Geometry: final body of the model. Coordinates: model frame, mm. Face numbers are marked on the shaded views. A direction names the side the tool comes from. Give positions to 0.01 mm unless a question says otherwise; leave off trailing zeros. Loops run counter-clockwise (first coordinate to the right, second up) from the corner with the lowest first, then second, coordinate; pieces in that order, holes last. Notation, with made-up numbers: (11.5, -32.5) -> (40.5, -32.5) arc R25 cw to (40.5, -0.5) -> close; hole circle Ø1 at (71.5, 68.25). An arc over 180 degrees is marked (long way). Answer in a Markdown table with one row per item. Add a question column.
1) Line query: line 1 (Y direction, x = -0.5, z = -9); line 2 (Z direction, x = 24, y = 9); line 3 (Z direction, x = 7, y = -8). Output: solid intervals per line, ascending. Write a range as from..to.
2) First-contact query: P1, Ø1, axis at x = -3.5, z = -2, coming from the -Y side; P2, Ø12, axis at y = 3.5, z = -1, coming from the +X side; P3, Ø6.5, axis at x = 25, z = 0, coming from the -Y side. Flat tips, straight axial feed; report the tip coordinate or a pass-through.
3) Draft query along Y for the marked faces 3, 4 and 5. Return one class per face: +Y half, -Y half, draft (parallel to the pull), parting line (faces both ways), or undercut.
4) Section query D-D (x = 25). Return the cut outline in (y, z).
5) Section query A-A (x = 9.5). Return the cut outline in (y, z).
6) Access query for the marked faces 1 and 2. Directions: +Z, -Z, +X, -X, +Y, -Y. A direction counts if a zero-diameter tool reaches every point of the face in a straight line with its end or side. Return the directions, or none.
```python
from build123d import *

# Parameters (mm, degrees)
SKETCH_1_W          = 60
SKETCH_1_H          = 45
EXTRUDE_1_DEPTH     = 13.5
CHAMFER_1_SIZE      = 10
FILLET_1_R          = 5
SHELL_1_T           = -1.5
FILLET_2_R          = 0.1
SKETCH_4_W          = 42
SKETCH_4_H          = 24
SKETCH_4_W_2        = 38
SKETCH_4_H_2        = 20
EXTRUDE_1_2_DEPTH   = 1
EXTRUDE_START       = 1
SKETCH_5_R          = 4
EXTRUDE_2_DEPTH     = 1
EXTRUDE_3_DEPTH     = 10
CUT_EXTRUDE_1_REACH = 47.349
SKETCH_7_R          = 2.5


with BuildPart() as part:
    # 草图1 → Extrude 1 (new, symmetric)
    with BuildSketch(Plane(origin=(0, 0, 0), x_dir=(1, 0, 0), z_dir=(0, 1, 0))):
        Rectangle(SKETCH_1_W, SKETCH_1_H)
    extrude(amount=EXTRUDE_1_DEPTH, both=True)

    # 倒角1
    chamfer_1_edges = [part.edges().sort_by_distance(p)[0] for p in [
        (-30, 0, 22.5),
        (-30, 0, -22.5),
    ]]
    chamfer(chamfer_1_edges, length=CHAMFER_1_SIZE)

    # 圆角1
    fillet_1_edges = [part.edges().sort_by_distance(p)[0] for p in [
        (-30, 0, 12.5),
        (-30, 0, -12.5),
        (-20, 0, -22.5),
        (-20, 0, 22.5),
    ]]
    fillet(fillet_1_edges, radius=FILLET_1_R)

    # 抽壳1
    shell_1_openings = [part.faces().sort_by_distance(p)[0] for p in [
        (30, 0, 0),
    ]]
    offset(amount=SHELL_1_T, openings=shell_1_openings, kind=Kind.INTERSECTION)

    # 圆角2
    fillet_2_edges = [part.edges().sort_by_distance(p)[0] for p in [
        (-25, 13.5, -17.5),
        (-30, 13.5, 0),
        (-25, 13.5, 17.5),
        (6.035533906, 13.5, 22.5),
        (-19.84234935, 13.5, 22.119397663),
        (-29.619397663, 13.5, 12.34234935),
        (-29.619397663, 13.5, -12.34234935),
        (-19.84234935, 13.5, -22.119397663),
        (-25, -13.5, -17.5),
        (-30, -13.5, 0),
        (6.035533906, -13.5, 22.5),
        (-25, -13.5, 17.5),
        (-19.84234935, -13.5, 22.119397663),
        (-29.619397663, -13.5, 12.34234935),
        (-29.619397663, -13.5, -12.34234935),
        (-19.84234935, -13.5, -22.119397663),
        (30, 13.5, 0),
        (6.035533906, -13.5, -22.5),
        (30, -12, 0),
        (30, 0, 21),
        (30, 0, -21),
        (30, 12, 0),
        (30, -13.5, 0),
        (6.035533906, 13.5, -22.5),
        (30, 0, 22.5),
        (30, 0, -22.5),
    ]]
    fillet(fillet_2_edges, radius=FILLET_2_R)

    # 草图3 → 旋转1 (revolve)
    with BuildSketch(Plane.XY, mode=Mode.PRIVATE) as revolve_1_sk:
        Polygon((0, 12), (4, 12), (4, 3.5), (14, 3.5), (14, 2.5), (12.5, 2.5), (12.5, -7.5), (14, -7.5), (14, -8.5), (4, -8.5), (4, -12), (0, -12), align=None)
    revolve(revolve_1_sk.sketch.rotate(Axis((0, 13.4, 0), (0, -1, 0)), 90), axis=Axis((0, 13.4, 0), (0, -1, 0)))

    # 草图4 → Extrude 1 2 (add, symmetric)
    with BuildSketch(Plane(origin=(20, 0, 0), x_dir=(0, 0, -1), z_dir=(1, 0, 0))):
        Rectangle(SKETCH_4_W, SKETCH_4_H)
        Rectangle(SKETCH_4_W_2, SKETCH_4_H_2, mode=Mode.SUBTRACT)
    extrude(amount=EXTRUDE_1_2_DEPTH, both=True)

    # 草图5 → 凸台-拉伸2 (add)
    with BuildSketch(Plane.XZ.offset(13.5).offset(EXTRUDE_START)):
        with Locations(Location((0, 0, 0), (0, 0, 90))):
            Circle(SKETCH_5_R)
    extrude(amount=-EXTRUDE_2_DEPTH)

    # 草图6 → 凸台-拉伸3 (add)
    with BuildSketch(Plane.XZ.offset(14.5)):
        Polygon((4, 0), (2, 3.464101615), (-2, 3.464101615), (-4, 0), (-2, -3.464101615), (2, -3.464101615), align=None)
    extrude(amount=EXTRUDE_3_DEPTH)

    # 草图7 → 切除-拉伸1 (cut, up to next)
    with BuildSketch(Plane(origin=(0, -12, 0), x_dir=(1, 0, 0), z_dir=(0, 1, 0)), mode=Mode.PRIVATE) as cut_extrude_1_sk1:
        with Locations(Location((25, 0, 0), (0, 0, 270))):
            Circle(SKETCH_7_R)
    cut_extrude_1_tool1 = extrude(cut_extrude_1_sk1.sketch, amount=-CUT_EXTRUDE_1_REACH, mode=Mode.PRIVATE) & part.part
    add(cut_extrude_1_tool1.solids().sort_by_distance((25, -12, 0))[0], mode=Mode.SUBTRACT)


solid = part.part
```
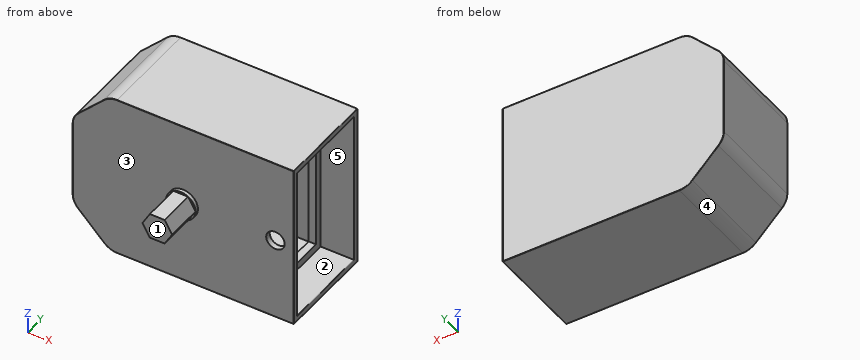
Evaluation:
| question | item | result |
|---|---|---|
| 1 | line 1 | -13.5..-12, -8.5..3.5, 12..13.5 |
| 1 | line 2 | -22.5..-21, 21..22.5 |
| 1 | line 3 | -22.5..-21, -12.12..12.12, 21..22.5 |
| 2 | P1 | y = -14.5 |
| 2 | P2 | x = 14 |
| 2 | P3 | y = -13.5 |
| 3 | face 3 | -Y half |
| 3 | face 4 | draft |
| 3 | face 5 | undercut |
| 4 | outline | (-13.5, -22.4) arc R0.1 ccw to (-13.4, -22.5) -> (13.4, -22.5) arc R0.1 ccw to (13.5, -22.4) -> (13.5, 22.4) arc R0.1 ccw to (13.4, 22.5) -> (-13.4, 22.5) arc R0.1 ccw to (-13.5, 22.4) -> (-13.5, 2.5) -> (-12, 2.5) -> (-12, 21) -> (12, 21) -> (12, -21) -> (-12, -21) -> (-12, -2.5) -> (-13.5, -2.5) -> close |
| 5 | outline | (-13.5, -22.4) arc R0.1 ccw to (-13.4, -22.5) -> (13.4, -22.5) arc R0.1 ccw to (13.5, -22.4) -> (13.5, 22.4) arc R0.1 ccw to (13.4, 22.5) -> (-13.4, 22.5) arc R0.1 ccw to (-13.5, 22.4) -> close; (-8.5, -10.28) -> (-7.5, -10.28) -> (-7.5, -8.12) -> (2.5, -8.12) -> (2.5, -10.28) -> (3.5, -10.28) -> (3.5, 10.28) -> (2.5, 10.28) -> (2.5, 8.12) -> (-7.5, 8.12) -> (-7.5, 10.28) -> (-8.5, 10.28) -> close; hole (-12, -21) -> (12, -21) -> (12, 21) -> (-12, 21) -> close |
| 6 | face 1 | +Z, -Z, +X, -X, -Y |
| 6 | face 2 | +X |
